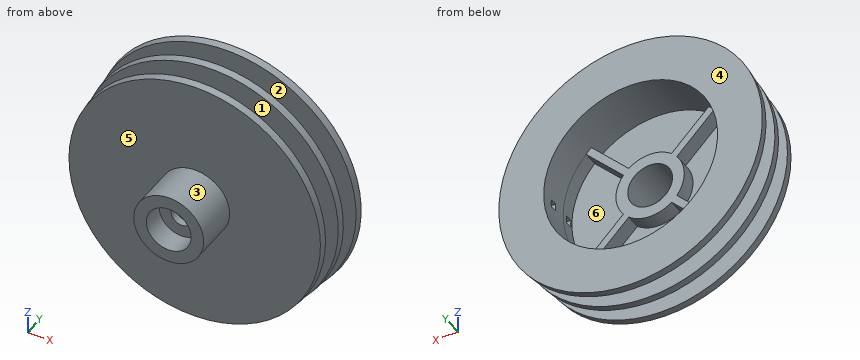
```python
from build123d import *
from build123d.topology import SkipClean

# Parameters (mm, degrees)
ESQUISSE2_R              = 2.95
ENL_V_MAT_EXTRU_1_DEPTH  = 3
ESQUISSE3_R              = 11.45
ENL_V_MAT_EXTRU_2_DEPTH  = 4.5
ENL_V_MAT_EXTRU_11_DEPTH = 2
ENL_V_START              = -5.5
ESQUISSE4_R              = 2.95
ENL_V_MAT_EXTRU_3_DEPTH  = 5.5
ESQUISSE6_R              = 1.4
ENL_V_MAT_EXTRU_9_DEPTH  = 27.496131793
ENL_V_START_2            = 5
ESQUISSE7_W              = 1
ESQUISSE7_H              = 1
ENL_V_MAT_EXTRU_10_DEPTH = 24.249690264


with BuildPart() as part:
    # Esquisse1 → Révolution1 (revolve)
    with BuildSketch(Plane.XY, mode=Mode.PRIVATE) as r_volution1_sk:
        Polygon((0, 0), (4.6, 0), (4.6, 6), (16.55, 6), (16.65, 7), (12.25, 7), (12.25, 9.5), (16.9, 9.5), (17, 10.5), (12.25, 10.5), (12.25, 13), (17.25, 13), (17.35, 14), (0, 14), align=None)
    revolve(r_volution1_sk.sketch.rotate(Axis((0, 0, 0), (0, 1, 0)), 90), axis=Axis((0, 0, 0), (0, 1, 0)))

    # Esquisse2 → Enlèv. mat.-Extru.1 (cut)
    with BuildSketch(Plane.XZ):
        with Locations(Location((0, 0, 0), (0, 0, 270))):
            Circle(ESQUISSE2_R)
    extrude(amount=-ENL_V_MAT_EXTRU_1_DEPTH, mode=Mode.SUBTRACT)

    # Esquisse3 → Enlèv. mat.-Extru.2 (cut)
    with BuildSketch(Plane(origin=(0, 14, 0), x_dir=(1, 0, 0), z_dir=(0, 1, 0))):
        with Locations(Location((0, 0, 0), (0, 0, 270))):
            Circle(ESQUISSE3_R)
    extrude(amount=-ENL_V_MAT_EXTRU_2_DEPTH, mode=Mode.SUBTRACT)

    # Esquisse8 → Enlèv. mat.-Extru.11 (cut)
    with SkipClean():  # the faces are left unmerged after this step: merging them gives an invalid solid
        with BuildSketch(Plane(origin=(0, 9.5, 0), x_dir=(1, 0, 0), z_dir=(0, 1, 0))):
            with BuildLine():
                Line((2.80872427, 3.515831051), (7.735096064, 8.442202845))
                ThreePointArc((7.735096064, 8.442202845), (0, 11.45), (-7.735096064, 8.442202845))
                Line((-7.735096064, 8.442202845), (-2.80872427, 3.515831051))
                ThreePointArc((-2.80872427, 3.515831051), (0, 4.5), (2.80872427, 3.515831051))
            make_face()
            with BuildLine():
                Line((3.515831051, 2.80872427), (8.442202845, 7.735096064))
                ThreePointArc((8.442202845, 7.735096064), (11.45, 0), (8.442202845, -7.735096064))
                Line((8.442202845, -7.735096064), (3.515831051, -2.80872427))
                ThreePointArc((3.515831051, -2.80872427), (4.5, 0), (3.515831051, 2.80872427))
            make_face()
            with BuildLine():
                Line((2.80872427, -3.515831051), (7.735096064, -8.442202845))
                ThreePointArc((7.735096064, -8.442202845), (0, -11.45), (-7.735096064, -8.442202845))
                Line((-7.735096064, -8.442202845), (-2.80872427, -3.515831051))
                ThreePointArc((-2.80872427, -3.515831051), (0, -4.5), (2.80872427, -3.515831051))
            make_face()
            with BuildLine():
                Line((-3.515831051, -2.80872427), (-8.442202845, -7.735096064))
                ThreePointArc((-8.442202845, -7.735096064), (-11.45, 0), (-8.442202845, 7.735096064))
                Line((-8.442202845, 7.735096064), (-3.515831051, 2.80872427))
                ThreePointArc((-3.515831051, 2.80872427), (-4.5, 0), (-3.515831051, -2.80872427))
            make_face()
        extrude(amount=-ENL_V_MAT_EXTRU_11_DEPTH, mode=Mode.SUBTRACT)

    # Esquisse4 → Enlèv. mat.-Extru.3 (cut)
    with SkipClean():  # the faces are left unmerged after this step: merging them gives an invalid solid
        with BuildSketch(Plane(origin=(0, 9.5, 0), x_dir=(1, 0, 0), z_dir=(0, 1, 0)).offset(ENL_V_START)):
            with Locations(Location((0, 0, 0), (0, 0, 90))):
                Circle(ESQUISSE4_R)
        extrude(amount=ENL_V_MAT_EXTRU_3_DEPTH, mode=Mode.SUBTRACT)

    # Esquisse6 → Enlèv. mat.-Extru.9 (cut, through all)
    with SkipClean():  # the faces are left unmerged after this step: merging them gives an invalid solid
        with BuildSketch(Plane(origin=(0, 4, 0), x_dir=(1, 0, 0), z_dir=(0, 1, 0))):
            with Locations(Location((0, 0, 0), (0, 0, 270))):
                Circle(ESQUISSE6_R)
        extrude(amount=-ENL_V_MAT_EXTRU_9_DEPTH, mode=Mode.SUBTRACT)

    # Esquisse7 → Enlèv. mat.-Extru.10 (cut, through all)
    with BuildSketch(Plane(origin=(0, 0, 0), x_dir=(0, 0, -1), z_dir=(1, 0, 0)).offset(ENL_V_START_2)):
        with Locations((0, 11.75)):
            Rectangle(ESQUISSE7_W, ESQUISSE7_H)
        with Locations((0, 8.25)):
            Rectangle(ESQUISSE7_W, ESQUISSE7_H)
    extrude(amount=ENL_V_MAT_EXTRU_10_DEPTH, mode=Mode.SUBTRACT)


solid = part.part
```
The listing builds one solid part. Answer for the finished solid, in the listing's coordinates (mm). Face numbers are marked on the shaded views. A direction names the side the tool comes from. Coordinates: 2 decimals unless noted, no trailing zeros. Write each loop counter-clockwise with the first axis right and the second up, starting at its lowest first coordinate (ties: lowest second). Pieces come first, ordered by that corner, then holes. Notation, with made-up numbers: (9, 4.25) - (45, 4.25) arc R15 cw to (45, 20.25) - close; hole circle Ø9 at (55.5, 28). An arc over 180 degrees is marked (long way). Return JSON: item names as keys, results as strings. Group by question number.
1. A cutting plane is placed at B-B, the plane y = 5.5. Determine the outline of the cut face in (x, z), plus the area to 3 significant figures.
2. A cutting plane is placed at A-A, the plane z = 0. Give the number of separate pieces and of enclosed holes in the cut face, plus the area to 3 significant figures.
3. Given pin 1 (1.5 mm diameter, centred on x = -8.5, z = 10, fed in from -Y); pin 2 (3 mm diameter, centred on x = -12.5, y = 5, fed in from -Z); pin 3 (3 mm diameter, centred on y = 12, z = -6.5, fed in from +X); pin 4 (8.5 mm diameter, centred on x = 2, z = -8, fed in from +Y), each flat-ended and moving along its own axis, determine where each tip first touches the part or whether it passes through.
4. Which of the six approach directions +Z, -Z, +X, -X, +Y, -Y give full straight-line access (tool end or side, diameter ignored) to the marked faces 5 and 6?
5. Straight lines are drawn through the part: L1, parallel to X at y = 9.25, z = 0; L2, parallel to Y at x = -10, z = 9.5; L3, parallel to X at y = 8, z = -6. For each, find the intervals that lie inside material, in ascending order.
6. Determine the mould class of the marked faces 1, 2, 3 and 4 for opening direction Y: released by +Y, released by -Y, zero draft, split by the parting line, or undercut.
Ans:
{
 "1": {"outline": "circle Ø9.2 at (0, 0); hole circle Ø5.9 at (0, 0)", "area": "39.1 mm²"},
 "2": {"separate pieces": "4", "enclosed holes": "0", "area": "94.0 mm²"},
 "3": {"pin 1": "y = 6", "pin 2": "z = -12.01", "pin 3": "x = 16.39", "pin 4": "y = 14"},
 "4": {"face 5": "-Y", "face 6": "+Y"},
 "5": {"L1": "-12.25 to -11.45, -4.5 to -2.95, 2.95 to 4.5, 11.45 to 12.25", "L2": "6 to 7, 9.5 to 10.5, 13 to 14", "L3": "-10.68 to -9.75, -6.71 to -5.29, 5.29 to 6.71, 9.75 to 10.68"},
 "6": {"face 1": "undercut", "face 2": "undercut", "face 3": "zero draft", "face 4": "released by +Y"}
}
